Study the drawing (mm; zero at the part's minimum x, y, z) and answer. A direction names the side the tool comes from. Coordinates: 2 decimals unless noted, no trailing zeros. Loops run counter-clockwise (first coordinate to the right, second up) from the corner with the lowest first, then second, coordinate; pieces in that order, holes last. Notation, with made-up numbers: M -5,5 L 10,5 A24 ccw 10,24 Z; hole C 8.25,15 d8. An arc over 180 degrees is marked long. Use one line per item in the form item = value. Start each with the question number.
1. The part is cut by section D-D (x = 40). Give the vertices of the cut face in (y, z).
2. The part is cut by section A-A (y = 25.5). Give the vertices of the cut face in (x, z).
3. The part is cut by section C-C (z = 1.7). Give the vertices of the cut face in (x, y).
4. The part is cut by section B-B (x = 22.75). Give the vertices of the cut face in (y, z), plus the area to 3 significant figures.
5. For a pull along Y with two mould halves and no side action, classify the marked faces 1, 2 and 3 as released by +Y, released by -Y, zero draft, split by the parting line, or undercut.
6. A flat-ended cylindrical pin translates along its axis: pin 1 (2 mm diameter, centred on x = 25, z = 1.5, fed in from -Y). Find the tip coordinate at first contact, or state that the pin passes through.
7. A tool of negligible diameter and unlimited length cuts with its end or side. For the marked faces 4, 5 and 6, from which of +Z, -Z, +X, -X, +Y, -Y can it reach the whole face along a straight path? Write none if from no direction.
8. Find the intervals of material crossed by probe 1 along Y at (x, z) = (22.75, 1.85); probe 2 along Y at (x, z) = (8.5, 2.6); probe 3 along X at (y, z) = (28, 1.75), in increasing order. Write a range as [from, to].
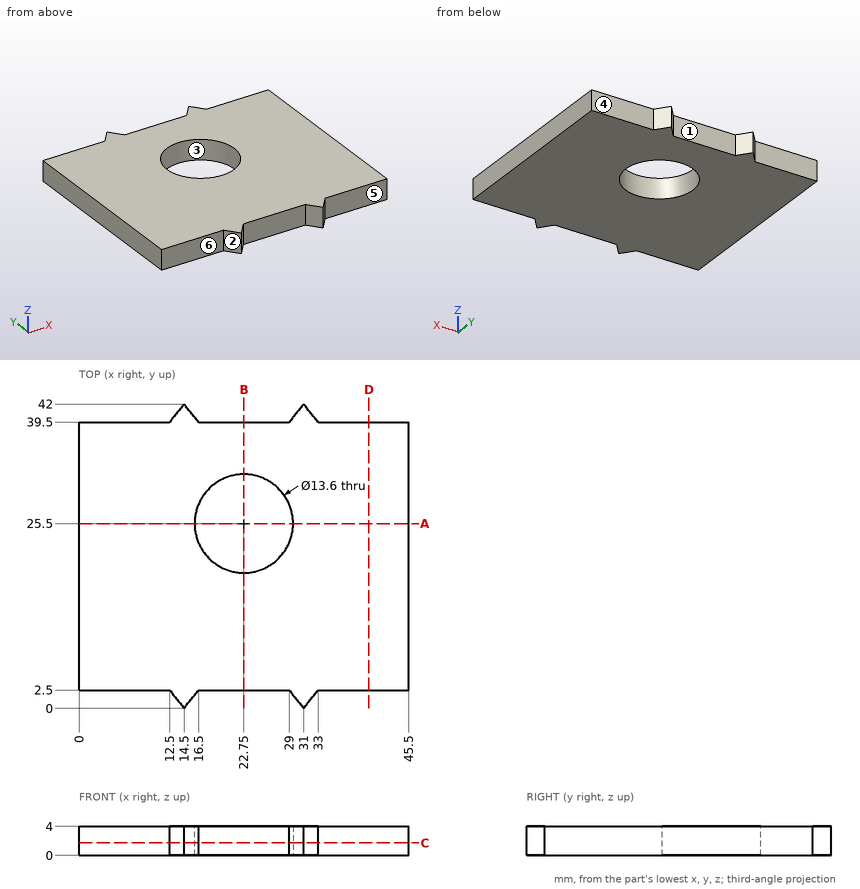
Computed values:
q1.outline = M 2.5,0 L 39.5,0 L 39.5,4 L 2.5,4 Z
q2.outline = M 0,0 L 15.95,0 L 15.95,4 L 0,4 Z; M 29.55,0 L 45.5,0 L 45.5,4 L 29.55,4 Z
q3.outline = M 0,2.5 L 12.5,2.5 L 14.5,0 L 16.5,2.5 L 29,2.5 L 31,0 L 33,2.5 L 45.5,2.5 L 45.5,39.5 L 33,39.5 L 31,42 L 29,39.5 L 16.5,39.5 L 14.5,42 L 12.5,39.5 L 0,39.5 Z; hole C 22.75,25.5 d13.6
q4.outline = M 2.5,0 L 18.7,0 L 18.7,4 L 2.5,4 Z; M 32.3,0 L 39.5,0 L 39.5,4 L 32.3,4 Z
q4.area = 93.6 mm²
q5.face_1 = released by +Y
q5.face_2 = released by -Y
q5.face_3 = undercut
q6.pin_1 = 2.5
q7.face_4 = +Z, -Z, +X, +Y
q7.face_5 = +Z, -Z, +X, -Y
q7.face_6 = +Z, -Z, -X, -Y
q8.probe_1 = [2.5, 18.7], [32.3, 39.5]
q8.probe_2 = [2.5, 39.5]
q8.probe_3 = [0, 16.43], [29.07, 45.5]
